Verification items for the finished model (mm, model axes). Round coordinates to 2 decimals unless told otherwise and drop trailing zeros. Order: outer loops, then holes, each group sorted by start corner. A loop starts at its lowest first (then second) coordinate and runs counter-clockwise, first axis right, second up. Notation, with made-up numbers: (18.25, 66.25) -> (33.25, 66.25) arc R30 ccw to (33.25, 93.25) -> close; hole circle Ø1 at (-12.5, -32.5). An arc over 180 degrees is marked (long way). Return JSON: item names as keys, results as strings. Group by question number.
Item 1: Scan lines: probe 1 along Z at (x, y) = (-10, 3.3); probe 2 along X at (y, z) = (2, -47.5); probe 3 along X at (y, z) = (1, -145). Record each from-to range of solid material in increasing order. Write a range as from..to.
Item 2: Sectioned sample at D-D on z = -145. Record the cut outline in (x, y), plus the area to 4 significant figures.
Item 3: Depth check by flat-ended pin: pin 1 Ø4.5 at (x, z) = (-115, -47.5) entering from +Y. Enter the tip coordinate at first touch or a pass-through.
Item 4: Sectioned sample at A-A on x = -95. Record the cut outline in (y, z).
Item 5: Sectioned sample at B-B on x = -40. Record the cut outline in (y, z).
Item 6: Sectioned sample at C-C on z = -85. Record the cut outline in (x, y).
Item 7: Draft check along Z on faces 1 (the cylindrical face through (-1, 3, -168)), 2 (the cylindrical face through (-8.73, 2.54, -142.56)), 3 (the flat face through (-74, 5, -84)). Enter one of: pulls with the +Z half, pulls with the -Z half, needs draft (parallel to the pull), parting line crosses it, or undercut.
Autodesk Inventor part; units mm, degrees
ref_plane "YZ Plane" through (0, 0, 0) normal (1, 0, 0) x (0, 1, 0)
ref_plane "XZ Plane" through (0, 0, 0) normal (0, 1, 0) x (-1, 0, 0)
ref_plane "XY Plane" through (0, 0, 0) normal (0, 0, 1) x (1, 0, 0)
sketch "Sketch1" plane through (0, 0, 0) normal (0, 1, 0) x (-1, 0, 0)
  line L0 (0, 0) -> (150, 0)
  line L1 (150, 0) -> (150, -170)
  line L2 (150, -170) -> (0, -170)
  line L3 (0, -170) -> (0, 0)
  dimension "d0" = 150
  dimension "d1" = 170
extrude "Extrusion1" add sketch "Sketch1" along normal blind 5
fillet "Fillet1" radius 5 4 edges at (0, 2.5, 0) (0, 2.5, -170) (-150, 2.5, 0) (-150, 2.5, -170)
sketch "Sketch2" plane through (0, 5, 0) normal (0, 1, 0) x (1, 0, 0)
  arc A0 (-145, 170) -> (-150, 165) centre (-145, 165) ccw
  line L0 (-150, 165) -> (-150, 5)
  arc A1 (-150, 5) -> (-145, 0) centre (-145, 5) ccw
  line L1 (-145, 0) -> (-5, 0)
  arc A2 (-5, 0) -> (0, 5) centre (-5, 5) ccw
  line L2 (0, 5) -> (0, 165)
  arc A3 (0, 165) -> (-5, 170) centre (-5, 165) ccw
  line L3 (-5, 170) -> (-145, 170)
  circle A4 centre (-125, 145) radius 2.75
  circle A5 centre (-140.5, 160.5) radius 1.75
  circle A6 centre (-140.5, 129.5) radius 1.75
  circle A7 centre (-109.5, 160.5) radius 1.75
  circle A8 centre (-109.5, 129.5) radius 1.75
  circle A9 centre (-40, 25) radius 2.75
  circle A10 centre (-10, 25) radius 2.75
  circle A11 centre (-40, 145) radius 2.75
  circle A12 centre (-10, 145) radius 2.75
  circle A13 centre (-10, 85) radius 2.75
  circle A14 centre (-40, 70) radius 2.75
  circle A15 centre (-40, 100) radius 2.75
  circle A16 centre (-115, 47.5) radius 2.75
  circle A17 centre (-95, 47.5) radius 2.75
  point P0 (0, 0)
  dimension "d5" = 5.5
  dimension "d6" = 25
  dimension "d7" = 25
  dimension "d8" = 3.5
  dimension "d9" = 9.5
  dimension "d10" = 9.5
  dimension "d13" = 31
  dimension "d16" = 31
  dimension "d19" = 5.5
  dimension "d20" = 25
  dimension "d21" = 5.5
  dimension "d22" = 25
  dimension "d23" = 5.5
  dimension "d24" = 5.5
  dimension "d25" = 25
  dimension "d26" = 25
  dimension "d27" = 5.5
  dimension "d28" = 170
  dimension "d29" = 85
  dimension "d30" = 5.5
  dimension "d31" = 5.5
  dimension "d32" = 30
  dimension "d33" = 70
  dimension "d34" = 10
  dimension "d35" = 10
  dimension "d36" = 10
  dimension "d37" = 40
  dimension "d38" = 40
  dimension "d39" = 40
  dimension "d40" = 40
  dimension "d43" = 5.5
  dimension "d44" = 5.5
  dimension "d45" = 45
  dimension "d46" = 22.5
  dimension "d47" = 22.5
  dimension "d48" = 20
  dimension "d49" = 35
extrude "Extrusion2" cut sketch "Sketch2" against normal blind 5 contours A4 | A5 | A6 | A7 | A8 | A9 | A10 | A11 | A12 | A13 | A14 | A15 | A16 | A17
equation "\"d20\" = d6"
equation "\"d22\" = d20"
equation "\"d25\" = d6"
equation "\"d26\" = d25"
equation "\"d29\" = 0.5 * d28"
equation "\"d33\" = 0.5 * d28 - 0.5 * d32"
equation "\"d35\" = d34"
equation "\"d36\" = d34"
equation "\"d38\" = d37"
equation "\"d39\" = d38"
equation "\"d40\" = d37"
equation "\"d46\" = 0.5 * d45"
equation "\"d47\" = d46"
properties part number "HeadPlate" material "Steel, Carbon"
Recorded:
{
 "1": {"probe 1": "-170..-147.75, -142.25..-87.75, -82.25..-27.75, -22.25..0", "probe 2": "-150..-117.75, -112.25..-97.75, -92.25..0", "probe 3": "-150..-127.75, -122.25..-42.75, -37.25..-12.75, -7.25..0"},
 "2": {"outline": "(-150, 0) -> (-127.75, 0) -> (-127.75, 5) -> (-150, 5) -> close; (-122.25, 0) -> (-42.75, 0) -> (-42.75, 5) -> (-122.25, 5) -> close; (-37.25, 0) -> (-12.75, 0) -> (-12.75, 5) -> (-37.25, 5) -> close; (-7.25, 0) -> (0, 0) -> (0, 5) -> (-7.25, 5) -> close", "area": "667.5 mm²"},
 "3": {"pin 1": "through"},
 "4": {"outline": "(0, -170) -> (5, -170) -> (5, -50.25) -> (0, -50.25) -> close; (0, -44.75) -> (5, -44.75) -> (5, 0) -> (0, 0) -> close"},
 "5": {"outline": "(0, -170) -> (5, -170) -> (5, -147.75) -> (0, -147.75) -> close; (0, -142.25) -> (5, -142.25) -> (5, -102.75) -> (0, -102.75) -> close; (0, -97.25) -> (5, -97.25) -> (5, -72.75) -> (0, -72.75) -> close; (0, -67.25) -> (5, -67.25) -> (5, -27.75) -> (0, -27.75) -> close; (0, -22.25) -> (5, -22.25) -> (5, 0) -> (0, 0) -> close"},
 "6": {"outline": "(-150, 0) -> (-12.75, 0) -> (-12.75, 5) -> (-150, 5) -> close; (-7.25, 0) -> (0, 0) -> (0, 5) -> (-7.25, 5) -> close"},
 "7": {"face 1": "pulls with the -Z half", "face 2": "undercut", "face 3": "needs draft"}
}
